Here's how the part is built. I have some questions about the finished solid (model axes, mm). A direction names the side the tool comes from. Round coordinates to 2 decimals unless told otherwise and drop trailing zeros. Order: outer loops, then holes, each group sorted by start corner. A loop starts at its lowest first (then second) coordinate and runs counter-clockwise, first axis right, second up. Notation, with made-up numbers: (-20, 18) - (17, 18) arc R16 ccw to (17, 35) - close; hole circle Ø10 at (-13.75, 48.25). An arc over 180 degrees is marked (long way). Answer as a JSON object with one key per item and string values.
Autodesk Inventor part; units mm, degrees
ref_plane "YZ Plane" through (0, 0, 0) normal (1, 0, 0) x (0, 1, 0)
ref_plane "XZ Plane" through (0, 0, 0) normal (0, 1, 0) x (-1, 0, 0)
ref_plane "XY Plane" through (0, 0, 0) normal (0, 0, 1) x (1, 0, 0)
sketch "Sketch1" plane through (0, 0, 0) normal (0, 1, 0) x (-1, 0, 0)
  circle A0 centre (0, 0) radius 30
  circle A1 centre (0, 20.5) radius 8.75
  circle A2 centre (-17.7535, 10.25) radius 8.75
  circle A3 centre (-17.7535, -10.25) radius 8.75
  circle A4 centre (0, -20.5) radius 8.75
  circle A5 centre (17.7535, -10.25) radius 8.75
  circle A6 centre (17.7535, 10.25) radius 8.75
  circle A7 centre (20.5, 0) radius 7.5
  circle A8 centre (14.4957, 14.4957) radius 7.5
  circle A9 centre (0, 20.5) radius 7.5
  circle A10 centre (-14.4957, 14.4957) radius 7.5
  circle A11 centre (-20.5, 0) radius 7.5
  circle A12 centre (-14.4957, -14.4957) radius 7.5
  circle A13 centre (0, -20.5) radius 7.5
  circle A14 centre (14.4957, -14.4957) radius 7.5
  dimension "d0" = 60
  dimension "d19" = 17.5
  dimension "d20" = 20.5
  dimension "d23" = 360
  dimension "d25" = 15
  dimension "d26" = 20.5
  dimension "d29" = 360
extrude "Extrusion1" add sketch "Sketch1" along normal blind 8 contours A0 | A1 A8 A10 | A10 A1 | A1 A10 A2 | A8 A6 A1 | A1 A8 | A1 A8 A6 A7 A5 A14 A4 A12 A3 A11 A2 A10 | A10 A2 A11 | A2 A10 | A8 A6 | A6 A7 A8 | A11 A2 | A2 A11 A3 | A11 A3 A12 | A3 A11 | A7 A6 | A6 A7 A5 | A12 A3 | A3 A12 A4 | A7 A5 A14 | A5 A7 | A12 A4 A14 | A4 A12 | A14 A5 | A5 A14 A4 | A4 A14 | A9 | A13
sketch "Sketch2" plane through (0, 8, 0) normal (0, 1, 0) x (1, 0, 0)
  circle A0 centre (0, -20.5) radius 8.75
  line L0 (-8.75, -20.5) -> (-8.75, -28.6956)
  line L1 (8.75, -20.5) -> (8.75, -28.6956)
  circle A1 centre (0, 0) radius 30
  dimension "d3" = 17.5
  dimension "d4" = 20.5
extrude "Extrusion2" cut sketch "Sketch2" against normal blind 1.4 contours A0 | L1 A1 L0 A0 picked at (-5.5585, -28.7503)
sketch "Sketch3" plane through (0, 6.6, 20.5) normal (0, 1, 0) x (-1, 0, 0)
  arc A0 (-8.75, 0) -> (8.75, 0) centre (0, 0) ccw
  circle A1 centre (0, 0) radius 8
  line L0 (8, 0) -> (8, 8.4137)
  line L1 (-8, 0) -> (-8, 8.4137)
  arc A2 (8.75, 8.1956) -> (-8.75, 8.1956) centre (0, -20.5) ccw
  dimension "d7" = 16
extrude "Extrusion3" cut sketch "Sketch3" against normal through all
pattern_circular "Circular Pattern1" count 6 over 360 about axis through (0, 0, 0) along (0, 1, 0) of "Extrusion2", "Extrusion3"
sketch "Sketch7" plane through (0, 8, 0) normal (0, 1, 0) x (1, 0, 0)
  arc A0 (8, -20.5) -> (-8, -20.5) centre (0, -20.5) ccw
  circle A1 centre (0, -20.5) radius 8.75
  arc A2 (-13.7535, -17.1782) -> (-21.7535, -3.3218) centre (-17.7535, -10.25) ccw
  circle A3 centre (-17.7535, -10.25) radius 8.75
  line L0 (-21.04, -21.385) -> (-13.7535, -17.1782)
  line L1 (-8, -28.9137) -> (-8, -20.5)
  line L2 (-8, -24.0444) -> (-16.823, -18.9504)
  arc A4 (-20.4761, -21.9255) -> (-8.75, -28.6956) centre (0, 0) ccw
  arc A5 (-21.04, -21.385) -> (-20.4761, -21.9255) centre (0, 0) ccw
  arc A6 (-8.75, -28.6956) -> (-8, -28.9137) centre (0, 0) ccw
  dimension "d32" = 17.5
  dimension "d33" = 17.5
extrude "Extrusion6" cut sketch "Sketch7" against normal blind 10 contours L1 A6 A4 A5 L0 L2
pattern_circular "Circular Pattern2" count 6 over 360 about axis through (0, -10, 0) along (0, 1, 0) of "Extrusion6"
sketch "Sketch4" plane through (0, 8, 0) normal (0, 1, 0) x (1, 0, 0)
  circle A0 centre (0, 0) radius 3.5
  dimension "d13" = 7
extrude "Extrusion4" cut sketch "Sketch4" against normal through all
sketch "Sketch8" plane through (0, 8, 0) normal (0, 1, 0) x (1, 0, 0)
  circle A0 centre (0, 0) radius 9.5
  dimension "d39" = 19
extrude "Extrusion7" cut sketch "Sketch8" against normal blind 6
properties part number "motor_3DPrint"
1. Imagine slicing it at B-B (x = 0). List the corners of the cut face in (y, z) for me.
Responses:
{"outline": "(0, -12.5) - (6.6, -12.5) - (6.6, -11.75) - (8, -11.75) - (8, -9.5) - (2, -9.5) - (2, -3.5) - (0, -3.5) - close; (0, 3.5) - (2, 3.5) - (2, 9.5) - (8, 9.5) - (8, 11.75) - (6.6, 11.75) - (6.6, 12.5) - (0, 12.5) - close"}
2. If I drill on L1, parallel to Z at x = 0, y = 1.45; L2, parallel to Z at x = -10.5, y = 2.25; L3, parallel to Z at x = -12, y = 3, over which ranges is the centre line in solid material (lowest first)? Write a range as [from, to].
Responses:
{"L1": "[-12.5, -3.5], [3.5, 12.5]", "L2": "[-22.6, -13.62], [-6.88, 6.88], [13.62, 22.6]", "L3": "[-21.73, -15.81], [-4.69, 4.69], [15.81, 21.73]"}
3. Imagine slicing it at C-C (z = 10.25). List the corners of the cut face in (x, y) for me, plus the area to 3 significant figures.
Responses:
{"outline": "(-9.75, 0) - (9.75, 0) - (9.75, 6.6) - (9, 6.6) - (9, 8) - (-9, 8) - (-9, 6.6) - (-9.75, 6.6) - close", "area": "154 mm2"}
4. Imagine slicing it at A-A (y = 4). List the corners of the cut face in (x, z) for me.
Responses:
{"outline": "(-24.82, -5.09) - (-21.75, -3.32) arc R8 cw to (-13.75, -17.18) - (-16.82, -18.95) - (-8, -24.04) - (-8, -20.5) arc R8 cw to (8, -20.5) - (8, -24.04) - (16.82, -18.95) - (13.75, -17.18) arc R8 cw to (21.75, -3.32) - (24.82, -5.09) - (24.82, 5.09) - (21.75, 3.32) arc R8 cw to (13.75, 17.18) - (16.82, 18.95) - (8, 24.04) - (8, 20.5) arc R8 cw to (-8, 20.5) - (-8, 24.04) - (-16.82, 18.95) - (-13.75, 17.18) arc R8 cw to (-21.75, 3.32) - (-24.82, 5.09) - close; hole circle Ø19 at (0, 0)"}
5. Thinking about a two-plate mould opening in Z: for faces 5 (the face through (-14.707, 7.31, -18.595)), 6 (the face through (-0.192, 7.31, -11.752)), 7 (the face through (8.75, 7, 22)), which applies, pulls with the +Z half, pulls with the -Z half, needs draft (parallel to the pull), parting line crosses it, or undercut?
Responses:
{"face 5": "undercut", "face 6": "pulls with the -Z half", "face 7": "needs draft"}
6. Imagine slicing it at D-D (x = 18). List the corners of the cut face in (y, z) for me.
Responses:
{"outline": "(0, -2.25) - (6.6, -2.25) - (6.6, -1.5) - (8, -1.5) - (8, 1.5) - (6.6, 1.5) - (6.6, 2.25) - (0, 2.25) - close"}
7. For faces 1 (the face through (8, 3, 22)), 2 (the face through (14.707, 7.31, 18.595)), 3 (the face through (23.46, 7.31, 3.44)), 4 (the face through (10, 6.6, 7)), which set-ups out of +Z, -Z, +X, -X, +Y, -Y let a thin tool reach every point of the face, with its end or its side?
Responses:
{"face 1": "+Z, +Y, -Y", "face 2": "+X, +Y", "face 3": "+Z, +Y", "face 4": "+Y"}
8. For P1, Ø4, axis at y = 2.5, z = -21.5, coming from the +X side; P2, Ø4, axis at x = -13, z = 11, coming from the +Y side; P3, Ø0.7, axis at y = 7.5, z = -22, coming from the +X side; P4, Ø12.5, axis at x = -19, z = -6.5, coming from the +Y side, each with a flat end and sliding along its axis, tell me the tip position at first contact or that it passes through.
Responses:
{"P1": "x = 15.87", "P2": "through", "P3": "x = 12.15", "P4": "y = 8"}
